```python
from build123d import *

# Parameters (mm, degrees)
SKICA1_W                 = 40
SKICA1_H                 = 200
P_IDAT_VYSUNUT_M1_DEPTH  = 10
ZAOBLIT1_R               = 10
SKICA2_W                 = 12.7
SKICA2_H                 = 23.5
ODEBRAT_VYSUNUT_M1_DEPTH = 205.205778567


with BuildPart() as part:
    # Skica1 → Přidat vysunutím1 (new body)
    with BuildSketch(Plane.XY):
        with Locations((20, 100)):
            Rectangle(SKICA1_W, SKICA1_H)
    extrude(amount=P_IDAT_VYSUNUT_M1_DEPTH)

    # Zaoblit1
    zaoblit1_edges = [part.edges().sort_by_distance(p)[0] for p in [
        (0, 200, 5),
        (40, 200, 5),
        (40, 0, 5),
        (0, 0, 5),
    ]]
    fillet(zaoblit1_edges, radius=ZAOBLIT1_R)

    # Skica2 → Odebrat vysunutím1 (cut, through all)
    with BuildSketch(Plane.XY.offset(10)):
        with Locations((20, 178.25)):
            Rectangle(SKICA2_W, SKICA2_H)
    extrude(amount=-ODEBRAT_VYSUNUT_M1_DEPTH, mode=Mode.SUBTRACT)


solid = part.part
```
Check sheet for the modelled part. Datum: model origin and axes. Units: mm. A direction names the side the tool comes from. Give positions to 0.01 mm unless a question says otherwise; leave off trailing zeros. Order: outer loops, then holes, each group sorted by start corner. A loop starts at its lowest first (then second) coordinate and runs counter-clockwise, first axis right, second up. Notation, with made-up numbers: (-29, -34) -> (-12, -34) arc R20 cw to (-12, -28) -> close; hole circle Ø9 at (3.25, 25.25). An arc over 180 degrees is marked (long way). Return JSON: item names as keys, results as strings.
1. Cross-section at A-A, the plane x = 20.5. Record the cut outline in (y, z), plus the area to 4 significant figures.
From the geometry:
{"outline": "(0, 0) -> (166.5, 0) -> (166.5, 10) -> (0, 10) -> close; (190, 0) -> (200, 0) -> (200, 10) -> (190, 10) -> close", "area": "1,765 mm^2"}
2. Set-up check for faces 1 (the cylindrical face through (37.15, 196.99, 5.07)), 2 (the flat face through (20, 166.5, 5)): record each of +Z, -Z, +X, -X, +Y, -Y from which the full face is reachable in a straight line by a thin tool's end or side.
From the geometry:
{"face 1": "+Z, -Z, +X, +Y", "face 2": "+Z, -Z"}
3. Material ranges on probe 1 along Y at (x, z) = (21.5, 4); probe 2 along Y at (x, z) = (3.5, 3); probe 3 along Y at (x, z) = (9, 0.5), recorded low to high. Write a range as [from, to].
From the geometry:
{"probe 1": "[0, 166.5], [190, 200]", "probe 2": "[2.4, 197.6]", "probe 3": "[0.05, 199.95]"}
4. Cross-section at B-B, the plane y = 177. Record the cut outline in (x, z), plus the area to 3 significant figures.
From the geometry:
{"outline": "(0, 0) -> (13.65, 0) -> (13.65, 10) -> (0, 10) -> close; (26.35, 0) -> (40, 0) -> (40, 10) -> (26.35, 10) -> close", "area": "273 mm^2"}
5. Mould release check, pull along X, two halves, no side actions. Record for faces 3 (the flat face through (20, 101, 0)), 4 (the flat face through (13.65, 178, 5)), 5 (the flat face through (20, 190, 5)), 6 (the cylindrical face through (2.85, 3.01, 5.07)): +X half, -X half, draft (parallel to the pull), parting line (faces both ways), or undercut.
From the geometry:
{"face 3": "draft", "face 4": "undercut", "face 5": "undercut", "face 6": "-X half"}
6. Cross-section at C-C, the plane z = 5. Record the cut outline in (x, y), plus the area to 3 significant figures.
From the geometry:
{"outline": "(0, 10) arc R10 ccw to (10, 0) -> (30, 0) arc R10 ccw to (40, 10) -> (40, 190) arc R10 ccw to (30, 200) -> (10, 200) arc R10 ccw to (0, 190) -> close; hole (13.65, 166.5) -> (26.35, 166.5) -> (26.35, 190) -> (13.65, 190) -> close", "area": "7,620 mm^2"}
7. Cross-section at D-D, the plane x = 35.5. Record the cut outline in (y, z).
From the geometry:
{"outline": "(1.65, 0) -> (198.35, 0) -> (198.35, 10) -> (1.65, 10) -> close"}
